Print and shaded views of the part. All mm, measured from the part's lowest x, y and z. A direction names the side the tool comes from. Coordinates: 2 decimals unless noted, no trailing zeros. Loops run counter-clockwise (first coordinate to the right, second up) from the corner with the lowest first, then second, coordinate; pieces in that order, holes last.
1) Saw through at A-A, the plane y = 25. Write the cut outline in (x, z).
2) Saw through at B-B, the plane z = 34.5. Write the cut outline in (x, y).
3) Pin check, flat tips, straight feed: pin 1 Ø10 at (x, z) = (23, 16) entering from -Y; pin 2 Ø10 at (x, y) = (65, 23.5) entering from -Z; pin 3 Ø3 at (x, z) = (30, 40) entering from -Y. Stop position of each tip, or through.
4) Saw through at C-C, the plane x = 19.5. Write the cut outline in (y, z).
5) Two-plate mould, pull along Z, no slides. Class the marked faces 1, 2 and 3: +Z half, -Z half, draft (parallel to the pull), parting line (faces both ways), or undercut.
6) Wall check: line 1 along Z through (x, y) = (18, 36.5); line 2 along Y through (x, z) = (40, 40.5); line 3 along Z through (x, y) = (22, 34.5). Give the ranges that are in metal, low to high.
7) Which spindle directions (+Z, -Z, +X, -X, +Y, -Y) get a long thin tool onto all of the face, cutting with end or side? Do the marked faces 4 and 5. Say none if no direction does.
8) Saw through at D-D, the plane y = 17. Write the cut outline in (x, z).
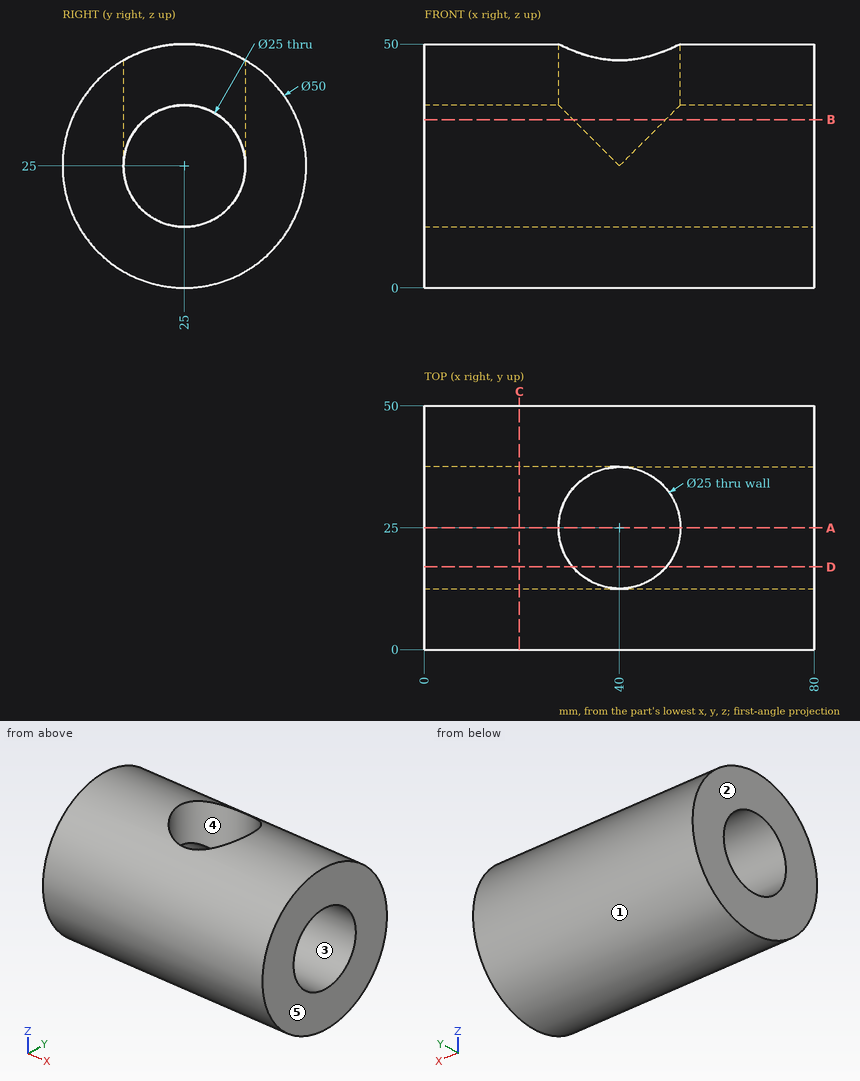
Data:
1. outline: (0, 0) - (80, 0) - (80, 12.5) - (0, 12.5) - close; (0, 37.5) - (27.5, 37.5) - (27.5, 50) - (0, 50) - close; (52.5, 37.5) - (80, 37.5) - (80, 50) - (52.5, 50) - close
2. outline: (0, 1.88) - (80, 1.88) - (80, 16.88) - (49.5, 16.88) arc R12.5 cw to (30.5, 16.88) - (0, 16.88) - close; (0, 33.12) - (30.5, 33.12) arc R12.5 cw to (49.5, 33.12) - (80, 33.12) - (80, 48.12) - (0, 48.12) - close
3. pin 1: stops at y = 0.32
3. pin 2: stops at z = 0
3. pin 3: stops at y = 3.96
4. outline: circle Ø50 at (25, 25); hole circle Ø25 at (25, 25)
5. face 1: parting line
5. face 2: draft
5. face 3: undercut
6. line 1: z = 2.8 to 20.1, 29.9 to 47.2
6. line 2: y = 5.38 to 12.5, 37.5 to 44.62
6. line 3: z = 1.88 to 16.88, 33.12 to 48.12
7. face 4: +Z
7. face 5: +Z, -Z, +X, +Y, -Y
8. outline: (0, 1.31) - (80, 1.31) - (80, 15.4) - (0, 15.4) - close; (0, 34.6) - (30.4, 34.6) - (30.4, 48.69) - (0, 48.69) - close; (49.6, 34.6) - (80, 34.6) - (80, 48.69) - (49.6, 48.69) - close
